Can you work these out from the model? Positions are in its coordinate system, mm. A direction names the side the tool comes from. Round coordinates to 2 decimals unless told otherwise and drop trailing zeros. Loops run counter-clockwise (first coordinate to the right, second up) from the corner with the lowest first, then second, coordinate; pieces in that order, holes last.
from build123d import *

# Parameters (mm, degrees)
BOSS_EXTRUDE1_DEPTH = 3
BOSS_EXTRUDE3_DEPTH = 17


with BuildPart() as part:
    # Sketch1 → Boss-Extrude1 (new body)
    with BuildSketch(Plane(origin=(0, 0, 0), x_dir=(0, 0, -1), z_dir=(1, 0, 0))):
        Polygon((0, 0), (-12.814351741, 0), (0.221356727, 5.4), (1.606108813, 5), (16.606108813, 30.980762114), (18.91550989, 30.980762114), (3.585414012, 4.428257168), (18.91550989, 0), align=None)
    boss_extrude1 = extrude(amount=BOSS_EXTRUDE1_DEPTH)

    # Sketch3 → Boss-Extrude3 (add)
    with BuildSketch(Plane(origin=(20, 0, 0), x_dir=(0, 0, -1), z_dir=(1, 0, 0))):
        Polygon((3.585414012, 4.428257168), (1.606108813, 5), (3.106108813, 7.598076211), (5.085414012, 7.026333379), align=None)
    boss_extrude3 = extrude(amount=-BOSS_EXTRUDE3_DEPTH)

    # Mirror5: Boss-Extrude3 across plane
    add(boss_extrude3.mirror(Plane(origin=(20, 0, 0), x_dir=(0, 0, 1), z_dir=(1, 0, 0))))

    # Mirror6: Boss-Extrude1 across plane
    add(boss_extrude1.mirror(Plane(origin=(20, 0, 0), x_dir=(0, 0, 1), z_dir=(1, 0, 0))))


solid = part.part
(1) Will these pins go through, and if not, where does the flat tip stop? P1, Ø8, axis at x = 26, y = 3.5, coming from the +Z side; P2, Ø8, axis at y = 7, z = 8, coming from the -X side.
Worked answers:
P1: stops at z = -1.61
P2: passes through
(2) If we mould it in two halves opening along Z, with no side actions, what happens to faces 1 (the flat face through (38.52, 2.66, 6.39)), 2 (the flat face through (1, 30.981, -18)), 3 (the flat face through (38.521, 5.203, -0.904))? For each: released by +Z, released by -Z, zero draft, split by the parting line, or undercut.
Worked answers:
face 1: released by +Z
face 2: zero draft
face 3: undercut
(3) If we section it at D-D, the plane x = 19: List the corners of the cut face in (y, z) for me, then the cut area to 3 significant figures.
Worked answers:
outline: (4.43, -3.59) - (7.03, -5.09) - (7.6, -3.11) - (5, -1.61) - close
area: 6.00 mm2
(4) If we section it at B-B, the plane y = 21: List the corners of the cut face in (x, z) for me, then the cut area to 3 significant figures.
Worked answers:
outline: (0, -13.15) - (3, -13.15) - (3, -10.84) - (0, -10.84) - close; (37, -13.15) - (40, -13.15) - (40, -10.84) - (37, -10.84) - close
area: 13.9 mm2
(5) If we section it at C-C, the plane z = 2: List the corners of the cut face in (x, y) for me, then the cut area to 3 significant figures.
Worked answers:
outline: (0, 0) - (3, 0) - (3, 4.48) - (0, 4.48) - close; (37, 0) - (40, 0) - (40, 4.48) - (37, 4.48) - close
area: 26.9 mm2
(6) If we section it at A-A, the plane z = -10.5: List the corners of the cut face in (x, y) for me, then the cut area to 3 significant figures.
Worked answers:
outline: (0, 0) - (3, 0) - (3, 2.43) - (0, 2.43) - close; (0, 16.4) - (3, 16.4) - (3, 20.4) - (0, 20.4) - close; (37, 0) - (40, 0) - (40, 2.43) - (37, 2.43) - close; (37, 16.4) - (40, 16.4) - (40, 20.4) - (37, 20.4) - close
area: 38.6 mm2
(7) If I drill on line 1 (X direction, y = 18.5, z = -11.5); line 2 (Z direction, x = 24.5, y = 6), over which ranges is the centre line in solid material (lowest first)?
Worked answers:
line 1: x = 0 to 3, 37 to 40
line 2: z = -4.49 to -2.18
(8) For faces 4 (the flat face through (19.76, 4.71, -2.61)), 5 (the flat face through (19.762, 7.316, -4.082)), 6 (the flat face through (1.479, 2.245, -11.143)), 7 (the flat face through (1.479, 5.203, -0.904)), which set-ups out of +Z, -Z, +X, -X, +Y, -Y let a thin tool reach every point of the face, with its end or its side?
Worked answers:
face 4: +Z, -Y
face 5: -Z, +Y
face 6: -Z, +X, -X
face 7: +X, -X, +Y
